from build123d import *

# Parameters (mm, degrees)
F1_DEPTH  = 15.24
F4_DEPTH  = 25.4
F5_W      = 2.5342174816
F5_H      = 10.4648
F5_W_2    = 2.6317641129
F6_DEPTH  = 25.4
F8_DEPTH  = 25.4
F9_W      = 32.1324085817
F9_H      = 9.3754695263
F10_DEPTH = 25.4


with BuildPart() as f1:
    # F0 (on Front) → F1 (new body)
    with BuildSketch(Plane.XZ):
        with BuildLine():
            ThreePointArc((-47.0203304827, 93.7563699834), (-51.5104585433, 91.896498044), (-53.3703304827, 87.4063699834))
            Line((-53.3703304827, 87.4063699834), (-53.3703304827, 75.7731699834))
            Line((-53.3703304827, 75.7731699834), (-53.3703304827, -40.7366300166))
            ThreePointArc((-53.3703304827, -40.7366300166), (-51.5104585433, -45.2267580771), (-47.0203304827, -47.0866300166))
            Line((-47.0203304827, -47.0866300166), (11.4758695173, -47.0866300166))
            ThreePointArc((11.4758695173, -47.0866300166), (15.9659975778, -45.2267580771), (17.8258695173, -40.7366300166))
            Line((17.8258695173, -40.7366300166), (17.8258695173, 87.4063699834))
            ThreePointArc((17.8258695173, 87.4063699834), (15.9659975778, 91.896498044), (11.4758695173, 93.7563699834))
            Line((11.4758695173, 93.7563699834), (-47.0203304827, 93.7563699834))
        make_face()
    extrude(amount=F1_DEPTH)

    # F3 (on face) → F4 (cut)
    with BuildSketch(Plane.XZ.offset(15.24)):
        Polygon((10.6684593484, 87.0597213507), (-47.2460240126, 87.0597213507), (10.6684593484, -37.9136353731), align=None)
        Polygon((10.6684593484, -37.9136353731), (-47.2460240126, 87.0597213507), (-47.2460240126, -35.696811974), align=None)
        Polygon((-47.2460240126, -37.9136353731), (10.6684593484, -37.9136353731), (-47.2460240126, -35.696811974), align=None)
    extrude(amount=-F4_DEPTH, mode=Mode.SUBTRACT)

    # F5 (on face) → F6 (cut)
    with BuildSketch(Plane(origin=(-53.3703304827, 0, 0), x_dir=(0, -1, 0), z_dir=(-1, 0, 0))):
        with Locations((8.8871087408, 48.3919699834)):
            Rectangle(F5_W, F5_H)
        with Locations((6.3041179436, 48.3919699834)):
            Rectangle(F5_W_2, F5_H)
    extrude(amount=-F6_DEPTH, mode=Mode.SUBTRACT)

    # F7 (on face) → F8 (cut)
    with BuildSketch(Plane.YZ.offset(17.8258695173)):
        Polygon((-2.3553799838, 66.2608699834), (-7.62, 66.2608699834), (-11.4997718483, 66.2608699834), (-11.4997718483, 45.7714051008), (-2.3553799838, 45.7714051008), align=None)
    extrude(amount=-F8_DEPTH, mode=Mode.SUBTRACT)

    # F9 (on face) → F10 (cut)
    with BuildSketch(Plane(origin=(0, 0, -47.0866300166), x_dir=(1, 0, 0), z_dir=(0, 0, -1))):
        with Locations((-19.3419498391, 6.8665045546)):
            Rectangle(F9_W, F9_H)
    extrude(amount=-F10_DEPTH, mode=Mode.SUBTRACT)


solid = f1.part
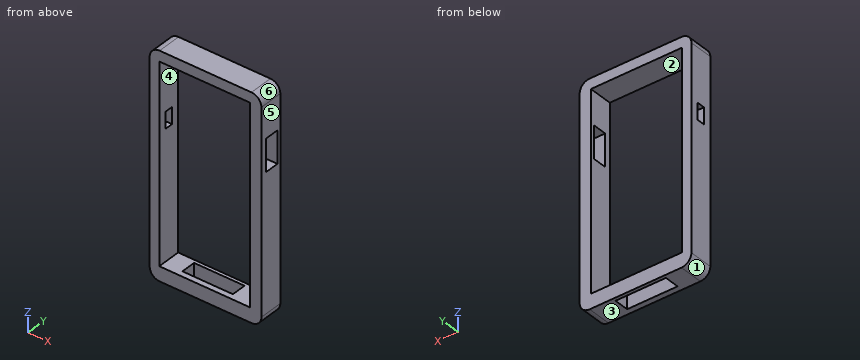
The model under review builds one solid part; all positions refer to its coordinate system, in mm. Face numbers are marked on the shaded views. A direction names the side the tool comes from. Round coordinates to 2 decimals unless told otherwise and drop trailing zeros. Loops run counter-clockwise (first coordinate to the right, second up) from the corner with the lowest first, then second, coordinate; pieces in that order, holes last. Notation, with made-up numbers: (-20.5, 74.5) -> (21.5, 74.5) arc R34 ccw to (21.5, 107.5) -> close; hole circle Ø1 at (20.25, 69). An arc over 180 degrees is marked (long way). One line per question, with ' | ' between items. Start each with the question number.
Item 1: Add section D-D, the plane y = -13. Write out the cut boundary in (x, z), then the cut area to 3 significant figures.
Item 2: Machinability: for the marked faces 1 and 2, which of the approach directions +Z, -Z, +X, -X, +Y, -Y give a long, thin tool a straight path to every point of the face, cutting with its end or side? Answer none if there is none.
Item 3: Wall thickness on line 1 along X through (y, z) = (-1.75, 11); line 2 along Z through (x, y) = (-33, -12.5); line 3 along Z through (x, y) = (-7, -3.5): over which ranges is each line inside the solid? List them lowest first. Write a range as [from, to].
Item 4: Add section C-C, the plane x = 2. Write out the cut boundary in (y, z), then the cut area to 3 significant figures.
Item 5: Add section B-B, the plane z = 13.5. Write out the cut boundary in (x, y).
Item 6: For pin 1 (2 mm diameter, centred on x = 15, y = -9, fed in from +Z); pin 2 (2.5 mm diameter, centred on x = -51.5, y = -8, fed in from +Z); pin 3 (4.5 mm diameter, centred on x = -12.5, y = -5.5, fed in from -Z), all flat-tipped, find the tip position at first contact; note any pin that passes through.
Item 7: Draft analysis for pull direction Z (two halves, no side actions). For the marked faces 3, 4, 5 and 6, state which applies: +Z half, -Z half, draft (parallel to the pull), parting line (faces both ways), or undercut.
Item 8: Add section A-A, the plane x = -13. Write out the cut boundary in (y, z).
Return value:
1) outline: (-53.37, -40.74) arc R6.35 ccw to (-47.02, -47.09) -> (11.48, -47.09) arc R6.35 ccw to (17.83, -40.74) -> (17.83, 87.41) arc R6.35 ccw to (11.48, 93.76) -> (-47.02, 93.76) arc R6.35 ccw to (-53.37, 87.41) -> close; hole (-47.25, -37.91) -> (10.67, -37.91) -> (10.67, 87.06) -> (-47.25, 87.06) -> close | area: 2,760 mm2
2) face 1: -Z, -X, +Y, -Y | face 2: +Y, -Y
3) line 1: x = [-53.37, -47.25], [10.67, 17.83] | line 2: z = [-47.09, -37.91], [87.06, 93.76] | line 3: z = [87.06, 93.76]
4) outline: (-15.24, -47.09) -> (0, -47.09) -> (0, -37.91) -> (-15.24, -37.91) -> close; (-15.24, 87.06) -> (0, 87.06) -> (0, 93.76) -> (-15.24, 93.76) -> close | area: 242 mm2
5) outline: (-53.37, -15.24) -> (-47.25, -15.24) -> (-47.25, 0) -> (-53.37, 0) -> close; (10.67, -15.24) -> (17.83, -15.24) -> (17.83, 0) -> (10.67, 0) -> close
6) pin 1: stops at z = 93.23 | pin 2: stops at z = 92.87 | pin 3: stops at z = 87.06
7) face 3: -Z half | face 4: undercut | face 5: draft | face 6: +Z half
8) outline: (-15.24, -47.09) -> (-11.55, -47.09) -> (-11.55, -37.91) -> (-15.24, -37.91) -> close; (-15.24, 87.06) -> (0, 87.06) -> (0, 93.76) -> (-15.24, 93.76) -> close; (-2.18, -47.09) -> (0, -47.09) -> (0, -37.91) -> (-2.18, -37.91) -> close
